Autodesk Inventor part; units mm, degrees
ref_plane "YZ Plane" through (0, 0, 0) normal (1, 0, 0) x (0, 1, 0)
ref_plane "XZ Plane" through (0, 0, 0) normal (0, 1, 0) x (-1, 0, 0)
ref_plane "XY Plane" through (0, 0, 0) normal (0, 0, 1) x (1, 0, 0)
sketch "Boceto1" plane through (0, 0, 0) normal (0, 1, 0) x (-1, 0, 0)
  line L0 (5, 25) -> (-5, 25)
  line L1 (-5, 25) -> (-5, -25)
  line L2 (-5, -25) -> (5, -25)
  line L3 (5, -25) -> (5, 25)
  line L4 (5, 25) -> (-5, -25) construction
  line L5 (-5, 25) -> (5, -25) construction
  circle A0 centre (0, 20) radius 3
  circle A1 centre (0, -20) radius 3
  point P0 (0, 0)
  dimension "d0" = 10
  dimension "d1" = 50
  dimension "d2" = 6
  dimension "d3" = 6
  dimension "d4" = 5
  dimension "d5" = 5
extrude "Extrusión1" add sketch "Boceto1" along normal mid plane 5
fillet "Empalme1" radius 5 4 edges at (5, 0, 25) (-5, 0, 25) (5, 0, -25) (-5, 0, -25)
properties material "Titanio"
Can you work these out from the model? Positions are in its coordinate system, mm. Give positions to 0.01 mm unless a question says otherwise; leave off trailing zeros. Loops run counter-clockwise (first coordinate to the right, second up) from the corner with the lowest first, then second, coordinate; pieces in that order, holes last. Notation, with made-up numbers: (28, 75) -> (50, 75) arc R19 ccw to (50, 90) -> close; hole circle Ø3 at (78, -7.75). An arc over 180 degrees is marked (long way). Use one line per item in the form item = value.
1) If we section it at B-B (y = 2.05): Count the separate pieces of the cut face and the enclosed holes in it, plus the area to 3 significant figures.
Answers:
separate_pieces = 1
enclosed_holes = 2
area = 422 mm²
2) If we section it at C-C (z = 22): Please give me the cut outline in (x, y), plus the area to 3 significant figures.
Answers:
outline = (-4.58, -2.5) -> (-2.24, -2.5) -> (-2.24, 2.5) -> (-4.58, 2.5) -> close; (2.24, -2.5) -> (4.58, -2.5) -> (4.58, 2.5) -> (2.24, 2.5) -> close
area = 23.5 mm²
3) If we section it at D-D (z = -18): Please give me the cut outline in (x, y), plus the area to 3 significant figures.
Answers:
outline = (-5, -2.5) -> (-2.24, -2.5) -> (-2.24, 2.5) -> (-5, 2.5) -> close; (2.24, -2.5) -> (5, -2.5) -> (5, 2.5) -> (2.24, 2.5) -> close
area = 27.6 mm²
4) Will these pins go through, and if not, where does the flat tip stop? pin 1 (1.5 mm diameter, centred on x = 3.5, y = 1, fed in from -Z); pin 2 (1 mm diameter, centred on x = 1, y = -1.5, fed in from +Z) (3 decimals).
Answers:
pin_1 = -24.18
pin_2 = 24.975
5) If we section it at A-A (x = 1): Please give me the cut outline in (y, z).
Answers:
outline = (-2.5, -24.9) -> (2.5, -24.9) -> (2.5, -22.83) -> (-2.5, -22.83) -> close; (-2.5, -17.17) -> (2.5, -17.17) -> (2.5, 17.17) -> (-2.5, 17.17) -> close; (-2.5, 22.83) -> (2.5, 22.83) -> (2.5, 24.9) -> (-2.5, 24.9) -> close
6) I need wall thicknesses on line 1 along Z through (x, y) = (0, 1.05); line 2 along Z through (x, y) = (-1.5, 2.1); line 3 along X through (y, z) = (2.2, 19). Which ranges of each line are inside material? Lowest first, please.
Answers:
line_1 = -25 to -23, -17 to 17, 23 to 25
line_2 = -24.77 to -22.6, -17.4 to 17.4, 22.6 to 24.77
line_3 = -5 to -2.83, 2.83 to 5
7) We'd pull the mould along X, two halves only. Please class faces 1 (the face through (-5, 0, 0)), 2 (the face through (0, 2.5, 0)), 3 (the face through (0.65, -0.04, 22.93)), 4 (the face through (3, 0, 24)): released by +X, released by -X, zero draft, split by the parting line, or undercut.
Answers:
face_1 = released by -X
face_2 = zero draft
face_3 = undercut
face_4 = released by +X
